Can you work these out from the model? Positions are in its coordinate system, mm. A direction names the side the tool comes from. Give positions to 0.01 mm unless a question says otherwise; leave off trailing zeros. Write each loop counter-clockwise with the first axis right and the second up, starting at its lowest first coordinate (ties: lowest second). Pieces come first, ordered by that corner, then holes. Notation, with made-up numbers: (56.25, 10.5) -> (82.25, 10.5) arc R31 ccw to (82.25, 40.5) -> close; hole circle Ø1 at (52, 5.5). An arc over 180 degrees is marked (long way). One line per item, written item: value.
from build123d import *

# Parameters (mm, degrees)
F0_W     = 45
F0_H     = 20
F1_DEPTH = 20
F3_DEPTH = 18
F4_R     = 9.99999


# Not quite as in the source:
# - a fillet or chamfer is up to 0.001 mm smaller than in the source, because OpenCascade refuses the exact size


with BuildPart() as f1:
    # F0 (on Top) → F1 (new body)
    with BuildSketch(Plane.XY):
        Rectangle(F0_W, F0_H)
    extrude(amount=F1_DEPTH)

    # F2 (on face) → F3 (cut)
    with BuildSketch(Plane(origin=(0, 0, 0), x_dir=(1, 0, 0), z_dir=(0, 0, -1))):
        Polygon((2.6396454307, -4.572), (5.2792908615, 0), (2.6396454307, 4.572), (-2.6396454307, 4.572), (-5.2792908615, 0), (-2.6396454307, -4.572), align=None)
    extrude(amount=-F3_DEPTH, mode=Mode.SUBTRACT)

    # F4 (radius 10 in the source; OpenCascade refuses exactly that, so slightly less here)
    f4_edges = [f1.edges().sort_by_distance(p)[0] for p in [
        (22.5, -10, 10),
        (-22.5, -10, 10),
        (22.5, 10, 10),
        (-22.5, 10, 10),
    ]]
    fillet(f4_edges, radius=F4_R)


solid = f1.part
1) If we section it at B-B (y = 4): Write out the boundary of the cut face in (x, z).
Answer list:
outline: (-21.67, 0) -> (-2.97, 0) -> (-2.97, 18) -> (2.97, 18) -> (2.97, 0) -> (21.67, 0) -> (21.67, 20) -> (-21.67, 20) -> close
2) Will these pins go through, and if not, where does the flat tip stop? pin 1 (4 mm diameter, centred on x = 16, z = 3.5, fed in from -Y); pin 2 (1 mm diameter, centred on y = 2.5, z = 12.5, fed in from +X).
Answer list:
pin 1: stops at y = -9.89
pin 2: stops at x = 22.3
3) I need wall thicknesses on L1, parallel to Y at x = 0.5, z = 15.25; L2, parallel to X at y = -4, z = 1.25; L3, parallel to Z at x = 4, y = -1.25. Which ranges of each line are inside material? Lowest first, please.
Answer list:
L1: y = -10 to -4.57, 4.57 to 10
L2: x = -21.67 to -2.97, 2.97 to 21.67
L3: z = 18 to 20
4) If we section it at C-C (x = -4.5): Write out the boundary of the cut face in (y, z), and give its area (3 significant figures).
Answer list:
outline: (-10, 0) -> (-1.35, 0) -> (-1.35, 18) -> (1.35, 18) -> (1.35, 0) -> (10, 0) -> (10, 20) -> (-10, 20) -> close
area: 351 mm^2
5) For faces 1 (the face through (3.98, -2.25, 8.87)), 2 (the face through (0, 0, 20)), which set-ups out of +Z, -Z, +X, -X, +Y, -Y let a thin tool reach every point of the face, with its end or its side?
Answer list:
face 1: -Z
face 2: +Z, +X, -X, +Y, -Y
6) We'd pull the mould along Y, two halves only. Please class faces 3 (the face through (-19.65, -6.99, 10.14)), 4 (the face through (-19.65, 6.99, 10.14)), 5 (the face through (-3.94, -2.32, 8.87)): released by +Y, released by -Y, zero draft, split by the parting line, or undercut.
Answer list:
face 3: released by -Y
face 4: released by +Y
face 5: undercut
7) If we section it at D-D (x = -14.5): Write out the boundary of the cut face in (y, z), and give its area (3 significant figures).
Answer list:
outline: (-9.8, 0) -> (9.8, 0) -> (9.8, 20) -> (-9.8, 20) -> close
area: 392 mm^2
